Geometry: final body of the model. Coordinates: model frame, mm. Give positions to 0.01 mm unless a question says otherwise; leave off trailing zeros. Write each loop counter-clockwise with the first axis right and the second up, starting at its lowest first coordinate (ties: lowest second). Pieces come first, ordered by that corner, then holes. Notation, with made-up numbers: (76.5, 24) - (100.5, 24) arc R15 ccw to (100.5, 50) - close; hole circle Ø5 at (-13, -31.5). An arc over 180 degrees is marked (long way). One line per question, with ' | ' between items. Start each with the question number.
```python
from build123d import *

# Parameters (mm, degrees)
F1_DEPTH = 10
F2_R     = 0.49999


# Not quite as in the source:
# - a fillet or chamfer is up to 0.001 mm smaller than in the source, because OpenCascade refuses the exact size


with BuildPart() as f1:
    # F0 (on Top) → F1 (new body)
    with BuildSketch(Plane.XY):
        with BuildLine():
            Line((-3.4753119677, 1.4087961978), (-3.75, 0))
            ThreePointArc((-3.75, 0), (-3.4444328428, -1.4826943014), (-2.5775293913, -2.723755172))
            Line((-2.5775293913, -2.723755172), (-1.8901882203, -1.9974204595))
            ThreePointArc((-1.8901882203, -1.9974204595), (-1.0873091543, 2.5259174181), (2.75, 0))
            ThreePointArc((2.75, 0), (2.5549370113, -1.0172496587), (1.9974204595, -1.8901882203))
            Line((1.9974204595, -1.8901882203), (2.723755172, -2.5775293913))
            ThreePointArc((2.723755172, -2.5775293913), (3.4840050154, -1.3871586256), (3.75, 0))
            Line((3.75, 0), (3.4774126757, 1.4036028936))
            ThreePointArc((3.4774126757, 1.4036028936), (2.0974972168, 3.1085375059), (0, 3.75))
            ThreePointArc((0, 3.75), (-2.0951747252, 3.1101033537), (-3.4753119677, 1.4087961978))
        make_face()
        with BuildLine():
            Line((-2.4917121164, 6.4533979566), (-3.4753119677, 1.4087961978))
            ThreePointArc((-3.4753119677, 1.4087961978), (-2.0951747252, 3.1101033537), (0, 3.75))
            ThreePointArc((0, 3.75), (-1.8382729519, 4.5556704706), (-2.4917121164, 6.4533979566))
        make_face()
        with BuildLine():
            ThreePointArc((2.5, 6.25), (1.767766953, 4.482233047), (0, 3.75))
            ThreePointArc((0, 3.75), (2.0974972168, 3.1085375059), (3.4774126757, 1.4036028936))
            Line((3.4774126757, 1.4036028936), (2.4872564888, 6.5021014854))
            ThreePointArc((2.4872564888, 6.5021014854), (2.4968120896, 6.3762116833), (2.5, 6.25))
        make_face()
        with BuildLine():
            ThreePointArc((-2.4917121164, 6.4533979566), (-1.8382729519, 4.5556704706), (0, 3.75))
            ThreePointArc((0, 3.75), (1.767766953, 4.482233047), (2.5, 6.25))
            ThreePointArc((2.5, 6.25), (2.4968120896, 6.3762116833), (2.4872564888, 6.5021014854))
            ThreePointArc((2.4872564888, 6.5021014854), (2.3111850264, 7.2031126763), (1.9419288742, 7.8244561752))
            Line((1.9419288742, 7.8244561752), (1.1651573245, 7.1946737051))
            ThreePointArc((1.1651573245, 7.1946737051), (1.4138132809, 6.7511307281), (1.5, 6.25))
            ThreePointArc((1.5, 6.25), (-0.4879304654, 4.831576981), (-1.1825651479, 7.1727890718))
            Line((-1.1825651479, 7.1727890718), (-1.9709419132, 7.7879817863))
            ThreePointArc((-1.9709419132, 7.7879817863), (-2.3289694602, 7.1587910945), (-2.4917121164, 6.4533979566))
        make_face()
    extrude(amount=F1_DEPTH)

    # F2 (radius 0.5 in the source; OpenCascade refuses exactly that, so slightly less here)
    f2_edges = [f1.edges().sort_by_distance(p)[0] for p in [
        (-1.182565, 7.172789, 5),
        (1.165157, 7.194674, 5),
        (-1.890188, -1.99742, 5),
        (1.99742, -1.890188, 5),
        (-1.970942, 7.787982, 5),
        (1.941929, 7.824456, 5),
        (2.723755, -2.577529, 5),
        (-2.577529, -2.723755, 5),
    ]]
    fillet(f2_edges, radius=F2_R)


solid = f1.part
```
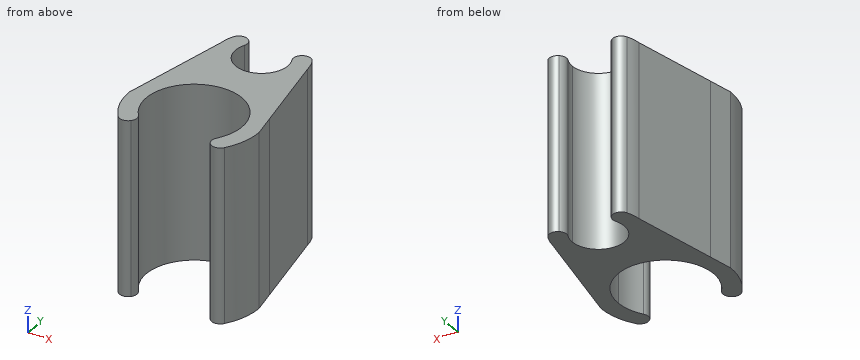
1) Section A-A, the plane y = 2. Output: boundary loops of the cut face in (x, z), plus the area to 3 significant figures.
2) Section B-B, the plane x = 0. Output: boundary loops of the cut face in (y, z).
3) First-contact query: pin 1 Ø1.5 at (x, z) = (-0.5, 1.5) entering from -Y; pin 2 Ø4 at (x, y) = (0, 3.5) entering from -Z; pin 3 Ø3 at (x, z) = (-1, 7) entering from +Y. Flat tips, straight axial feed; report the tip coordinate or a pass-through.
4) Line query: L1, parallel to X at y = 6.5, z = 1.25; L2, parallel to X at y = 2, z = 2; L3, parallel to Y at x = 0, z = 7.5. Output: solid intervals per line, ascending.
5) Section D-D, the plane y = -0.5. Output: boundary loops of the cut face in (x, z).
Answer key:
1) outline: (-3.36, 0) - (-1.89, 0) - (-1.89, 10) - (-3.36, 10) - close; (1.89, 0) - (3.36, 0) - (3.36, 10) - (1.89, 10) - close | area: 29.5 mm^2
2) outline: (2.75, 0) - (4.75, 0) - (4.75, 10) - (2.75, 10) - close
3) pin 1: y = 2.45 | pin 2: z = 0 | pin 3: y = 7.55
4) L1: -2.49 to -1.48, 1.48 to 2.49 | L2: -3.36 to -1.89, 1.89 to 3.36 | L3: 2.75 to 4.75
5) outline: (-3.72, 0) - (-2.7, 0) - (-2.7, 10) - (-3.72, 10) - close; (2.7, 0) - (3.72, 0) - (3.72, 10) - (2.7, 10) - close
